```python
from build123d import *

# Parameters (mm, degrees)
F0_W     = 69.85
F0_H     = 82.55
F1_DEPTH = 6.35
F2_W     = 82.55
F2_H     = 6.35
F3_ANGLE = -90
F4_W     = 6.35
F4_H     = 82.55
F5_DEPTH = 69.85


with BuildPart() as f1:
    # F0 (on Top) → F1 (new body)
    with BuildSketch(Plane.XY):
        with Locations((34.925, 41.275)):
            Rectangle(F0_W, F0_H)
    extrude(amount=F1_DEPTH)

    # F2 (on face) → F3 (revolve)
    with BuildSketch(Plane.YZ.offset(69.85)):
        with Locations((41.275, 3.175)):
            Rectangle(F2_W, F2_H)
    revolve(axis=Axis((69.85, 41.275, 6.35), (0, 1, 0)), revolution_arc=F3_ANGLE)

    # F4 (on face) → F5 (join)
    with BuildSketch(Plane.XY.offset(6.35)):
        with Locations((73.025, 41.275)):
            Rectangle(F4_W, F4_H)
    extrude(amount=F5_DEPTH)


solid = f1.part
```
Read the model definition and answer for the solid it produces. Units are mm, in the model's axes. A direction names the side the tool comes from. Coordinates: 2 decimals unless noted, no trailing zeros. Loops run counter-clockwise (first coordinate to the right, second up) from the corner with the lowest first, then second, coordinate; pieces in that order, holes last. Notation, with made-up numbers: (60.25, -6.75) - (92.25, -6.75) arc R9 ccw to (92.25, 10.25) - close; hole circle Ø3 at (27.5, 83). An arc over 180 degrees is marked (long way). Answer in a Markdown table with one row per item.
1. Find section C-C, the plane x = 62. Write down the section's boundary in (y, z), then the cut area to 3 significant figures.
Conclusion:
| item | result |
|---|---|
| outline | (0, 0) - (82.55, 0) - (82.55, 6.35) - (0, 6.35) - close |
| area | 524 mm² |
2. Given pin 1 (21 mm diameter, centred on x = 45.5, y = 49.5, fed in from +Z); pin 2 (4 mm diameter, centred on x = 68.5, z = 45, fed in from +Y); pin 3 (2 mm diameter, centred on y = 13.5, z = 50.5, fed in from -X), each flat-ended and moving along its own axis, determine where each tip first touches the part or whether it passes through.
Conclusion:
| item | result |
|---|---|
| pin 1 | stops at z = 6.35 |
| pin 2 | stops at y = 82.55 |
| pin 3 | stops at x = 69.85 |
3. Find section B-B, the plane z = 21. Write down the section's boundary in (x, y), then the cut area to 3 significant figures.
Conclusion:
| item | result |
|---|---|
| outline | (69.85, 0) - (76.2, 0) - (76.2, 82.55) - (69.85, 82.55) - close |
| area | 524 mm² |
4. Which of the six approach directions +Z, -Z, +X, -X, +Y, -Y give full straight-line access (tool end or side, diameter ignored) to faces 1 (the face through (0, 41, 3)), 2 (the face through (69.85, 41, 41))?
Conclusion:
| item | result |
|---|---|
| face 1 | +Z, -Z, -X, +Y, -Y |
| face 2 | +Z, -X, +Y, -Y |
5. Find section A-A, the plane y = 70. Write down the section's boundary in (x, z).
Conclusion:
| item | result |
|---|---|
| outline | (0, 0) - (69.85, 0) arc R6.35 ccw to (76.2, 6.35) - (76.2, 76.2) - (69.85, 76.2) - (69.85, 6.35) - (0, 6.35) - close |
6. Straight lines are drawn through the part: line 1 (Z direction, x = 58, y = 65); line 2 (X direction, y = 77.5, z = 60.5); line 3 (Z direction, x = 72, y = 62). For each, find the intervals that lie inside material, in ascending order.
Conclusion:
| item | result |
|---|---|
| line 1 | z = 0 to 6.35 |
| line 2 | x = 69.85 to 76.2 |
| line 3 | z = 0.38 to 76.2 |
